Geometry check sheet. Reference: drawing and pictorial views, mm from the part's lowest x, y, z. A direction names the side the tool comes from. Round coordinates to 2 decimals unless told otherwise and drop trailing zeros. Write each loop counter-clockwise with the first axis right and the second up, starting at its lowest first coordinate (ties: lowest second). Pieces come first, ordered by that corner, then holes. Notation, with made-up numbers: (-12.5, 24) - (25.5, 24) arc R26 cw to (25.5, 61) - close; hole circle Ø6 at (49.25, -28.75). An arc over 180 degrees is marked (long way). Use one line per item in the form item = value. Start each with the question number.
1) Section check B-B (x = 152.5). Record the boundary of the cut face in (y, z).
2) Gauge pin test, flat ends, axial feed: P1, Ø3, axis at x = 99.5, y = 55, coming from the -Z side; P2, Ø12, axis at x = 129.5, y = 90, coming from the +Z side; P3, Ø7, axis at y = 99, z = 26, coming from the +X side; P4, Ø1.5, axis at x = 108.5, y = 46.5, coming from the +Z side. Record the tip position at first contact, or that the pin passes through.
3) Scan lines: probe 1 along X at (y, z) = (57, 42); probe 2 along Y at (x, z) = (54, 50); probe 3 along Y at (x, z) = (105, 2). Record each from-to range of solid material in increasing order.
4) Section check A-A (z = 41). Record the boundary of the cut face in (x, y), then the cut area to 3 significant figures.
5) Section check C-C (y = 52). Record the boundary of the cut face in (x, z), then the cut area to 3 significant figures.
6) Set-up check for the marked faces 1 and 2: record each of +Z, -Z, +X, -X, +Y, -Y from which the full face is reachable in a straight line by a thin tool's end or side.
7) Section check D-D (x = 105). Record the boundary of the cut face in (y, z).
8) Draft check along X on the marked faces 3, 4 and 5. Enter one of: +X half, -X half, draft (parallel to the pull), parting line (faces both ways), or undercut.
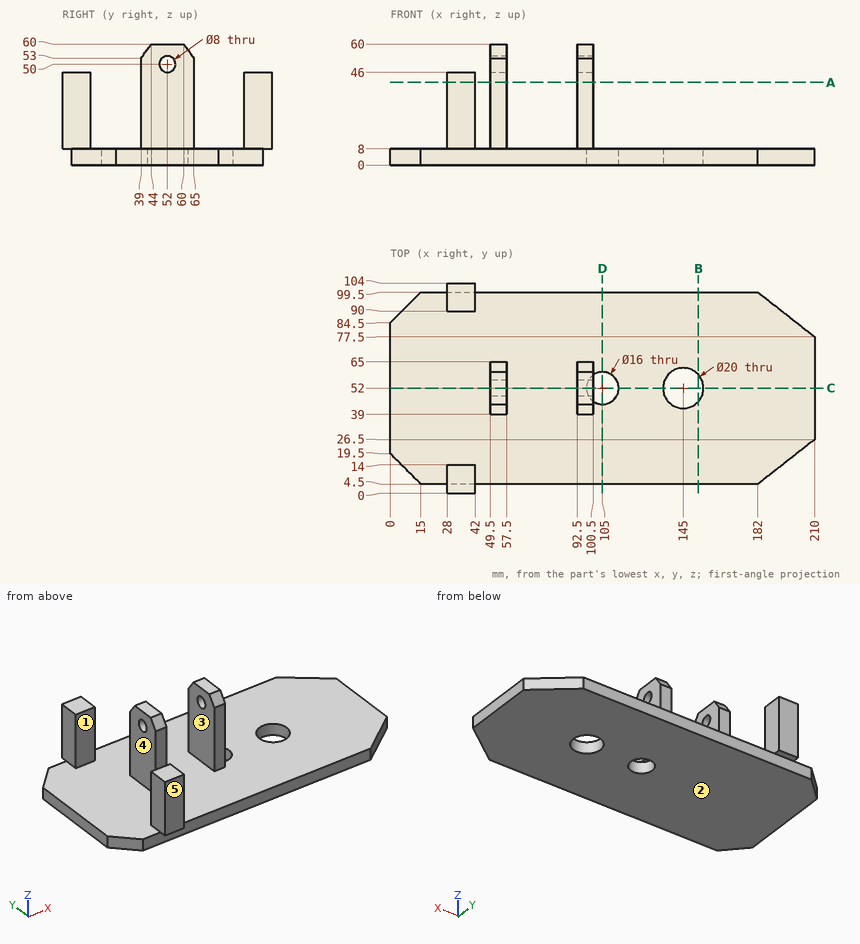
Results are:
q1.outline = (4.5, 0) - (45.39, 0) - (45.39, 8) - (4.5, 8) - close; (58.61, 0) - (99.5, 0) - (99.5, 8) - (58.61, 8) - close
q2.P1 = 8
q2.P2 = 8
q2.P3 = 42
q2.P4 = through
q3.probe_1 = 49.5 to 57.5, 92.5 to 100.5
q3.probe_2 = 39 to 48, 56 to 65
q3.probe_3 = 4.5 to 44, 60 to 99.5
q4.outline = (28, 0) - (42, 0) - (42, 14) - (28, 14) - close; (28, 90) - (42, 90) - (42, 104) - (28, 104) - close; (49.5, 39) - (57.5, 39) - (57.5, 65) - (49.5, 65) - close; (92.5, 39) - (100.5, 39) - (100.5, 65) - (92.5, 65) - close
q4.area = 808 mm²
q5.outline = (0, 0) - (97, 0) - (97, 8) - (100.5, 8) - (100.5, 46) - (92.5, 46) - (92.5, 8) - (57.5, 8) - (57.5, 46) - (49.5, 46) - (49.5, 8) - (0, 8) - close; (49.5, 54) - (57.5, 54) - (57.5, 60) - (49.5, 60) - close; (92.5, 54) - (100.5, 54) - (100.5, 60) - (92.5, 60) - close; (113, 0) - (135, 0) - (135, 8) - (113, 8) - close; (155, 0) - (210, 0) - (210, 8) - (155, 8) - close
q5.area = 2,100 mm²
q6.face_1 = +Z, +X, -X
q6.face_2 = -Z, +X, -X, +Y, -Y
q7.outline = (4.5, 0) - (44, 0) - (44, 8) - (4.5, 8) - close; (60, 0) - (99.5, 0) - (99.5, 8) - (60, 8) - close
q8.face_3 = undercut
q8.face_4 = -X half
q8.face_5 = draft
